Could you check a few things on this model? Use its own coordinates, in mm. Face numbers are marked on the shaded views. A direction names the side the tool comes from. Give positions to 0.01 mm unless a question says otherwise; leave off trailing zeros. Write each loop counter-clockwise with the first axis right and the second up, starting at its lowest first coordinate (ties: lowest second). Pieces come first, ordered by that corner, then holes. Notation, with made-up numbers: (12, -11.75) - (32, -11.75) arc R10 ccw to (32, -5.75) - close; hole circle Ø5 at (13.5, 0). An arc over 180 degrees is marked (long way). Answer in a Markdown table with one row per item.
Autodesk Inventor part; units mm, degrees
ref_plane "YZ Plane" through (0, 0, 0) normal (1, 0, 0) x (0, 1, 0)
ref_plane "XZ Plane" through (0, 0, 0) normal (0, 1, 0) x (-1, 0, 0)
ref_plane "XY Plane" through (0, 0, 0) normal (0, 0, 1) x (1, 0, 0)
sketch "Sketch1" plane through (0, 0, 0) normal (0, 1, 0) x (-1, 0, 0)
  circle A0 centre (0, 0) radius 1.225
  circle A1 centre (0, 0) radius 3.6287
  dimension "BoreD" = 2.45
  dimension "OuterD" = 7.2575
extrude "Extrusion1" add sketch "Sketch1" along normal blind 7
sketch "Sketch2" plane through (0, 0, 0) normal (0, -1, 0) x (1, 0, 0)
  circle A0 centre (0, 0) radius 3.6287
  arc A1 (0.4991, -3.4087) -> (0.6768, -3.5651) centre (0.6488, -3.4177) ccw
  arc A2 (0.4991, -3.4087) -> (-0.4991, -3.4087) centre (0, -3.3787) ccw
  arc A3 (-0.6768, -3.5651) -> (-0.4991, -3.4087) centre (-0.6488, -3.4177) ccw
  point P0 (0, -3.6287)
  dimension "d9" = 0.5
  dimension "d10" = 0.15
  dimension "Depth" = 0.25
extrude "Extrusion2" cut sketch "Sketch2" against normal up to next contours A3 A2 A1 A0 picked at (0, -3.374)
pattern_circular "Circular Pattern1" count 12 over 360 about axis through (0, -10, 0) along (0, 1, 0) of "Extrusion2"
sketch "Sketch3" plane through (0, 0, 0) normal (0, -1, 0) x (1, 0, 0)
  circle A0 centre (0, 0) radius 4.1287
  circle A1 centre (0, 0) radius 1.225
  dimension "FaceD" = 8.2575
  dimension "d18" = 2.45
extrude "Extrusion3" add sketch "Sketch3" along normal blind 1
equation "\"OuterD\" = 0.0604789 * Teeth"
equation "\"d18\" = BoreD"
equation "\"BeltWidth\" = 6"
equation "\"Pitch\" = 0.25"
properties part number "GT2 Gear"
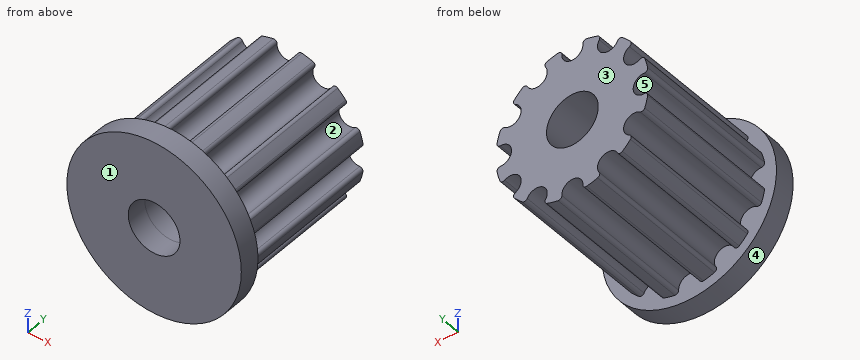
1) On a 3-axis mill with a long thin cutter (end or side, diameter ignored), from which of +Z, -Z, +X, -X, +Y, -Y can I reach the whole of each face in a straight line? I mean the marked faces 1 and 2. Say none if no direction works.
Check values:
| item | result |
|---|---|
| face 1 | +Z, -Z, +X, -X, -Y |
| face 2 | +Y |
2) Imagine slicing it at C-C (z = 2.25). List the corners of the cut face in (x, y) for me.
Check values:
| item | result |
|---|---|
| outline | (-3.46, -1) - (3.46, -1) - (3.46, 0) - (2.78, 0) - (2.78, 7) - (-2.78, 7) - (-2.78, 0) - (-3.46, 0) - close |
3) If I drill on line 1 (Z direction, x = 0, y = 5) (3 decimals); line 2 (Z direction, x = 0, y = -0.45) (3 decimals); line 3 (Y direction, x = 3, z = 0), over which ranges is the centre line in solid material (lowest first)?
Check values:
| item | result |
|---|---|
| line 1 | z = -2.879 to -1.225, 1.225 to 2.879 |
| line 2 | z = -4.129 to -1.225, 1.225 to 4.129 |
| line 3 | y = -1 to 0 |
4) Will these pins go through, and if not, where does the flat tip stop? P1, Ø3, axis at x = 0, z = 0, coming from the -Y side; P2, Ø1, axis at y = 1, z = 3, coming from the -X side.
Check values:
| item | result |
|---|---|
| P1 | stops at y = -1 |
| P2 | stops at x = -2.63 |
5) Imagine slicing it at B-B (x = 0). List the corners of the cut face in (y, z) for me (3 decimals).
Check values:
| item | result |
|---|---|
| outline | (-1, -4.129) - (0, -4.129) - (0, -2.879) - (7, -2.879) - (7, -1.225) - (-1, -1.225) - close; (-1, 1.225) - (7, 1.225) - (7, 2.879) - (0, 2.879) - (0, 4.129) - (-1, 4.129) - close |
6) We'd pull the mould along Z, two halves only. Please class the marked faces 3, 4 and 5: +Z half, -Z half, draft (parallel to the pull), parting line (faces both ways), or undercut.
Check values:
| item | result |
|---|---|
| face 3 | draft |
| face 4 | parting line |
| face 5 | undercut |
7) Imagine slicing it at D-D (x = 1.75). List the corners of the cut face in (y, z) for me, then the cut area to 3 significant figures.
Check values:
| item | result |
|---|---|
| outline | (-1, -3.74) - (0, -3.74) - (0, -2.43) - (7, -2.43) - (7, 2.43) - (0, 2.43) - (0, 3.74) - (-1, 3.74) - close |
| area | 41.5 mm2 |
8) Imagine slicing it at A-A (z = 0). List the corners of the cut face in (x, y) for me (3 decimals).
Check values:
| item | result |
|---|---|
| outline | (-4.129, -1) - (-1.225, -1) - (-1.225, 7) - (-2.879, 7) - (-2.879, 0) - (-4.129, 0) - close; (1.225, -1) - (4.129, -1) - (4.129, 0) - (2.879, 0) - (2.879, 7) - (1.225, 7) - close |
